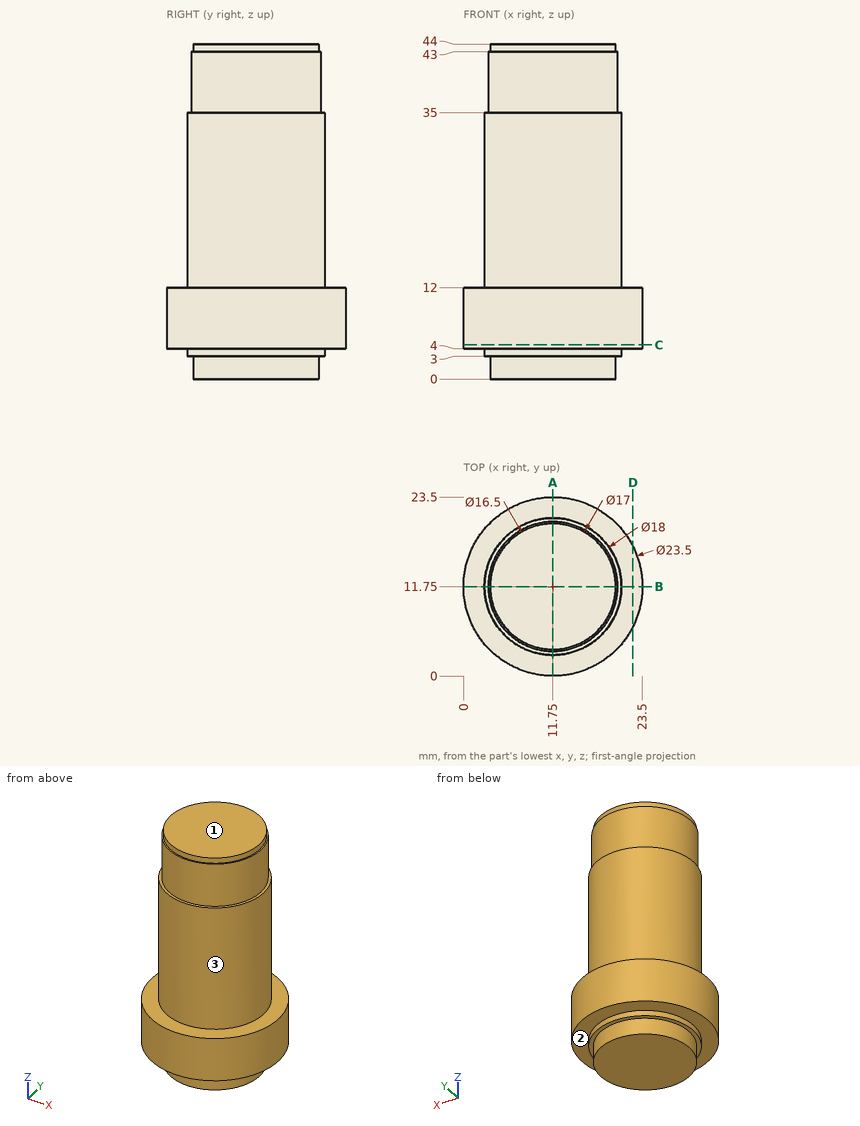
Source: three-view drawing plus pictorial views. Frame: mm from the lowest corner of the part. A direction names the side the tool comes from. Coordinates: 2 decimals unless noted, no trailing zeros. Order: outer loops, then holes, each group sorted by start corner. A loop starts at its lowest first (then second) coordinate and runs counter-clockwise, first axis right, second up. Notation, with made-up numbers: M 86,-28 L 100,-28 A18 ccw 100,-22 Z; hole C 81.5,16.5 d10. An arc over 180 degrees is marked long. Write each question's results on one line, items separated by ' | '. Start each with the question number.
1. Section C-C, the plane z = 4.5. Return the cut outline in (x, y).
2. Material intervals for L1, parallel to Z at x = 2.75, y = 6.75; L2, parallel to Y at x = 3.25, z = 10; L3, parallel to Y at x = 14.75, z = 13.5, sorted ascending.
3. Pin query (flat end, axial travel): pin 1 (6 mm diameter, centred on x = 18, z = 34, fed in from -Y); pin 2 (4 mm diameter, centred on x = 9, z = 6.5, fed in from -Y); pin 3 (1 mm diameter, centred on y = 7.5, z = 37.5, fed in from +X). Return the tip coordinate at first contact, or that it passes through.
4. Reachability of the marked faces 1, 2 and 3 from +Z, -Z, +X, -X, +Y, -Y: full face, straight path, thin tool, end or side. Return the list, or none.
5. Section A-A, the plane x = 11.75. Return the cut outline in (y, z), then the cut area to 3 significant figures.
6. Section D-D, the plane x = 22.25. Return the cut outline in (y, z).
Solution:
1) outline: C 11.75,11.75 d23.5
2) L1: 4 to 12 | L2: 3.64 to 19.86 | L3: 3.26 to 20.24
3) pin 1: y = 3.36 | pin 2: y = 0.02 | pin 3: x = 19.38
4) face 1: +Z, +X, -X, +Y, -Y | face 2: -Z | face 3: +Z
5) outline: M 0,4 L 2.75,4 L 2.75,3 L 3.5,3 L 3.5,0 L 20,0 L 20,3 L 20.75,3 L 20.75,4 L 23.5,4 L 23.5,12 L 20.75,12 L 20.75,35 L 20.25,35 L 20.25,43 L 20,43 L 20,44 L 3.5,44 L 3.5,43 L 3.25,43 L 3.25,35 L 2.75,35 L 2.75,12 L 0,12 Z | area: 822 mm²
6) outline: M 6.48,4 L 17.02,4 L 17.02,12 L 6.48,12 Z
